Check sheet for the modelled part. Datum: model origin and axes. Units: mm. A direction names the side the tool comes from. Round coordinates to 2 decimals unless told otherwise and drop trailing zeros. Loops run counter-clockwise (first coordinate to the right, second up) from the corner with the lowest first, then second, coordinate; pieces in that order, holes last. Notation, with made-up numbers: (89, 75) - (111, 75) arc R13 cw to (111, 81) - close; hole circle Ø7 at (48.25, -36.5). An arc over 180 degrees is marked (long way). Put each result on its own line as item: value. Start each with the question number.
```python
from build123d import *

# Parameters (mm, degrees)
F0_W     = 63.5
F0_H     = 19.05
F0_W_2   = 19.05
F1_DEPTH = 63.5
F0_W_3   = 25.4
F2_DEPTH = 25.4
F3_DEPTH = 7.9375
F5_R     = 6.35


with BuildPart() as f1:
    # F0 (on Front) → F1 (new body, symmetric)
    with BuildSketch(Plane.XZ):
        with Locations((-9.525, 0)):
            Rectangle(F0_W, F0_H)
        with Locations((31.75, 0)):
            Rectangle(F0_W_2, F0_H)
    extrude(amount=F1_DEPTH, both=True)

    # F0 (on Front) → F2 (join, symmetric)
    with BuildSketch(Plane.XZ):
        with BuildLine():
            Line((22.225, 9.525), (41.275, 9.525))
            Line((41.275, 9.525), (41.275, 27.004391))
            ThreePointArc((41.275, 27.004391), (45.79645, 38.1), (56.785241, 42.8752))
            Line((56.785241, 42.8752), (60.325, 42.8752))
            Line((60.325, 42.8752), (60.325, 61.9252))
            Line((60.325, 61.9252), (56.608955, 61.9252))
            ThreePointArc((56.608955, 61.9252), (32.263743, 51.508061), (22.225, 27.004391))
            Line((22.225, 27.004391), (22.225, 9.525))
        make_face()
        with Locations((73.025, 52.4002)):
            Rectangle(F0_W_3, F0_H)
    extrude(amount=F2_DEPTH, both=True)

    # F0 (on Front) → F3 (join, symmetric)
    with BuildSketch(Plane.XZ):
        with BuildLine():
            Line((-41.275, 9.525), (22.225, 9.525))
            Line((22.225, 9.525), (22.225, 27.004391))
            ThreePointArc((22.225, 27.004391), (32.263743, 51.508061), (56.608955, 61.9252))
            add(Edge.make_bspline(
                [(-41.275, 9.525), (-41.526487, 49.406126), (16.378682, 61.477449), (56.608955, 61.9252)],
                knots=[0, 0, 0, 0, 111.027247, 111.027247, 111.027247, 111.027247], degree=3))
        make_face()
    extrude(amount=F3_DEPTH, both=True)

    # F0 (on Front) → F4 (revolve)
    with BuildSketch(Plane.XZ):
        Polygon((85.725, 61.9252), (85.725, 42.8752), (85.725, 38.1), (111.125, 38.1), (111.125, 66.675), (85.725, 66.675), align=None)
    revolve(axis=Axis((85.725, 0, 52.3875), (0, 0, 1)))

    # F5
    f5_edges = [f1.edges().sort_by_distance(p)[0] for p in [
        (41.275, -63.5, 0),
        (-41.275, -63.5, 0),
        (41.275, 63.5, 0),
        (-41.275, 63.5, 0),
    ]]
    fillet(f5_edges, radius=F5_R)


solid = f1.part
```
Q1. Set-up check for faces 1 (the face through (45.7, -0.4, 38)), 2 (the face through (59, -2, 61.925)), 3 (the face through (32.532, -16.791, 51.778)), 4 (the face through (-4, 7.938, 30)), 5 (the face through (41.275, -1, 4)): record each of +Z, -Z, +X, -X, +Y, -Y from which the full face is reachable in a straight line by a thin tool's end or side.
Q2. Cross-section at C-C on y = -12.5. Enter the section's corners in (x, z) (3 decimals), and give its area (3 significant figures).
Q3. Cross-section at A-A on y = 38. Enter the section's corners in (x, z) (3 decimals).
Q4. Cross-section at B-B on x = 100.5. Enter the section's corners in (y, z) (3 decimals), and give its area (3 significant figures).
Q5. Depth check by flat-ended pin: pin 1 Ø12 at (x, y) = (-16.5, -37.5) entering from +Z (3 decimals); pin 2 Ø8 at (x, y) = (70.5, 25) entering from -Z; pin 3 Ø14 at (y, z) = (14.5, 20.5) entering from -X. Enter the tip coordinate at first touch or a pass-through.
Q6. Material ranges on line 1 (Z direction, x = 16, y = -15.5) (3 decimals); line 2 (Y direction, x = 12, z = 32.5); line 3 (Z direction, x = 99, y = -14) (3 decimals), recorded low to high. Write a range as from..to.
Answer list:
1. face 1: -Z, +Y, -Y
1. face 2: +Z, -X
1. face 3: +Z, -X, -Y
1. face 4: +Z, -X, +Y
1. face 5: -Z, +X, +Y, -Y
2. outline: (-41.275, -9.525) - (41.275, -9.525) - (41.275, 27.004) arc R15.875 cw to (56.785, 42.875) - (63.614, 42.875) - (63.614, 38.1) - (107.836, 38.1) - (107.836, 66.675) - (63.614, 66.675) - (63.614, 61.925) - (56.609, 61.925) arc R34.925 ccw to (22.225, 27.004) - (22.225, 9.525) - (-41.275, 9.525) - close
2. area: 4,050 mm2
3. outline: (-41.275, -9.525) - (41.275, -9.525) - (41.275, 9.525) - (-41.275, 9.525) - close
4. outline: (-20.661, 38.1) - (20.661, 38.1) - (20.661, 66.675) - (-20.661, 66.675) - close
4. area: 1,180 mm2
5. pin 1: stops at z = 9.525
5. pin 2: stops at z = 38.1
5. pin 3: stops at x = -40.38
6. line 1: z = -9.525..9.525
6. line 2: y = -7.94..7.94
6. line 3: z = 38.1..66.675
